Verification items for the finished model (mm, model axes). A direction names the side the tool comes from. Give positions to 0.01 mm unless a question says otherwise; leave off trailing zeros. Write each loop counter-clockwise with the first axis right and the second up, starting at its lowest first coordinate (ties: lowest second). Pieces come first, ordered by that corner, then holes. Notation, with made-up numbers: M 55.25,-11.5 L 90.25,-11.5 A27 cw 90.25,9.5 Z; hole C -34,-21.5 d6. An arc over 180 degrees is marked long. Write item = value, one per line.
from build123d import *

# Parameters (mm, degrees)
BOSS_EXTRUDE2_DEPTH = 88.9
CUT_EXTRUDE3_DEPTH  = 89.9
FILLET2_R           = 6.35
FILLET4_R           = 0.762


with BuildPart() as part:
    # Sketch1 → Boss-Extrude2 (new body)
    with BuildSketch(Plane.XY):
        Polygon((0, 0), (0, 101.6), (233.68, 101.6), (233.68, 88.9), (12.7, 88.9), (12.7, 0), align=None)
    extrude(amount=BOSS_EXTRUDE2_DEPTH)

    # Sketch8 → Cut-Extrude3 (cut, through all)
    with BuildSketch(Plane.XY.offset(88.9)):
        Polygon((228.6, 101.6), (233.68, 101.6), (233.68, 97.21103121), (232.101530561, 97.785547072), (231.371879071, 96.91598223), (230.178469436, 97.350347792), (230.178469436, 98.485484045), (228.6, 99.059999906), align=None)
        Polygon((228.6, 88.9), (233.68, 88.9), (233.68, 93.28896879), (232.101530561, 92.714452928), (231.371879071, 93.58401777), (230.178469436, 93.149652208), (230.178469436, 92.014515955), (228.6, 91.440000094), align=None)
    extrude(amount=-CUT_EXTRUDE3_DEPTH, mode=Mode.SUBTRACT)

    # Fillet2
    fillet2_edges = [part.edges().sort_by_distance(p)[0] for p in [
        (0, 101.6, 44.45),
        (12.7, 88.9, 44.45),
    ]]
    fillet(fillet2_edges, radius=FILLET2_R)

    # Fillet4
    fillet4_edges = [part.edges().sort_by_distance(p)[0] for p in [
        (228.6, 91.440000094, 44.45),
        (228.6, 99.059999906, 44.45),
    ]]
    fillet(fillet4_edges, radius=FILLET4_R)


solid = part.part
1) Cross-section at C-C on y = 20. Record the boundary of the cut face in (x, z).
From the geometry:
outline = M 0,0 L 12.7,0 L 12.7,88.9 L 0,88.9 Z
2) Cross-section at B-B on x = 140. Record the boundary of the cut face in (y, z).
From the geometry:
outline = M 88.9,0 L 101.6,0 L 101.6,88.9 L 88.9,88.9 Z
3) Tool access check on faces 1 (the flat face through (116, 101.6, 44)), 2 (the flat face through (125, 88.9, 44)). Record the directions out of +Z, -Z, +X, -X, +Y, -Y that give a thin tool (end or side, any length) a straight path to the whole face; none if there is none.
From the geometry:
face_1 = +Z, -Z, +X, -X, +Y
face_2 = +Z, -Z, +X, -Y
4) Material ranges on probe 1 along X at (y, z) = (12, 61); probe 2 along Y at (x, z) = (209, 74.5), recorded low to high. Write a range as from..to.
From the geometry:
probe_1 = 0..12.7
probe_2 = 88.9..101.6
5) Cross-section at A-A on z = 77. Record the boundary of the cut face in (x, y).
From the geometry:
outline = M 0,0 L 12.7,0 L 12.7,82.55 A6.35 cw 19.05,88.9 L 228.6,88.9 L 228.6,90.91 A0.76 cw 229.1,91.62 L 230.18,92.01 L 230.18,93.15 L 231.37,93.58 L 232.1,92.71 L 233.68,93.29 L 233.68,97.21 L 232.1,97.79 L 231.37,96.92 L 230.18,97.35 L 230.18,98.49 L 229.1,98.88 A0.76 cw 228.6,99.59 L 228.6,101.6 L 6.35,101.6 A6.35 ccw 0,95.25 Z
6) Depth check by flat-ended pin: P1, Ø2, axis at y = 89.5, z = 41, coming from the +X side; P2, Ø1, axis at x = 183, z = 60.5, coming from the -Y side; P3, Ø10, axis at x = 182.5, y = 87.5, coming from the -Z side; P4, Ø10, axis at y = 21, z = 74.5, coming from the +X side. Enter the tip coordinate at first touch or a pass-through.
From the geometry:
P1 = 228.6
P2 = 88.9
P3 = 0
P4 = 12.7
